Work out the finished part from the listing and answer in its coordinate system (mm). A direction names the side the tool comes from. Round coordinates to 2 decimals unless told otherwise and drop trailing zeros. Loops run counter-clockwise (first coordinate to the right, second up) from the corner with the lowest first, then second, coordinate; pieces in that order, holes last. Notation, with made-up numbers: M 6.25,-2 L 42.25,-2 A25 cw 42.25,20 Z; hole C 58,-17.5 d4. An arc over 180 degrees is marked long. One line per item, written item: value.
```python
from build123d import *

# Parameters (mm, degrees)
F2_SIZE2 = 10
F2_SIZE  = 10
F3_DEPTH = 25
F4_SIZE2 = 12
F4_SIZE  = 12


with BuildPart() as f1:
    # F0 (on Front) → F1 (revolve)
    with BuildSketch(Plane.XZ):
        Polygon((0, 40), (0, 0), (30, 0), (30, 25), (30, 40), align=None)
        with BuildLine():
            Line((30, 25), (30, 0))
            Line((30, 0), (96, 0))
            ThreePointArc((96, 0), (102, 6), (108, 0))
            Line((108, 0), (120, 0))
            Line((120, 0), (120, 25))
            Line((120, 25), (30, 25))
        make_face()
        with BuildLine():
            ThreePointArc((108, 0), (102, 6), (96, 0))
            Line((96, 0), (108, 0))
        make_face()
        with BuildLine():
            Line((108, 0), (96, 0))
            ThreePointArc((96, 0), (102, -6), (108, 0))
        make_face()
    revolve(axis=Axis((75, 0, 0), (1, 0, 0)))

    # F2
    f2_edges = [f1.edges().sort_by_distance(p)[0] for p in [
        (0, 0, -40),
    ]]
    chamfer(f2_edges, length=F2_SIZE, length2=F2_SIZE2)

    # F0 (on Front) → F3 (cut, symmetric)
    with BuildSketch(Plane.XZ):
        with BuildLine():
            ThreePointArc((108, 0), (102, 6), (96, 0))
            Line((96, 0), (108, 0))
        make_face()
        with BuildLine():
            Line((108, 0), (96, 0))
            ThreePointArc((96, 0), (102, -6), (108, 0))
        make_face()
    extrude(amount=F3_DEPTH, both=True, mode=Mode.SUBTRACT)

    # F4
    f4_edges = [f1.edges().sort_by_distance(p)[0] for p in [
        (120, 0, -25),
    ]]
    chamfer(f4_edges, length=F4_SIZE, length2=F4_SIZE2)


solid = f1.part
```
1) Each of these flat-tipped pins is pushed along its axis until it touches: pin 1 (3 mm diameter, centred on x = 105.5, z = 17, fed in from +Y); pin 2 (6 mm diameter, centred on y = 4.5, z = 22, fed in from +X); pin 3 (10 mm diameter, centred on x = 41.5, y = -13.5, fed in from +Z); pin 4 (8 mm diameter, centred on y = 15, z = -0.5, fed in from +X). Where does it stop, or does it pass through?
Check values:
pin 1: y = 19.62
pin 2: x = 113.54
pin 3: z = 23.51
pin 4: x = 120
2) The mould has two halves that part along Z. Classify faces 3 (the face through (0, 0, 0)), 4 (the face through (108, 0, 0)), 5 (the face through (0.49, -9.16, 29.08)): +Z half, -Z half, draft (parallel to the pull), parting line (faces both ways), or undercut.
Check values:
face 3: draft
face 4: undercut
face 5: parting line
3) Find the intervals of material crossed by probe 1 along X at (y, z) = (-1, 0); probe 2 along Z at (x, y) = (104, 20); probe 3 along Z at (x, y) = (102, 1.5), in increasing order. Write a range as from..to.
Check values:
probe 1: 0..96, 108..120
probe 2: -15..-5.66, 5.66..15
probe 3: -24.95..-6, 6..24.95
4) For faces 1 (the face through (19.86, 39.05, -8.67)), 2 (the face through (30, -18.34, -17.22)), determine the directions among +Z, -Z, +X, -X, +Y, -Y from which every point of the face is accessible in a straight line to the end or side of a thin tool.
Check values:
face 1: +X, -X
face 2: +X
5) Find section B-B (x = 88.5). Give the vertices of the cut face in (y, z), then the cut area to 3 significant figures.
Check values:
outline: C 0,0 d50
area: 1,960 mm2
6) Find section A-A (y = 0). Give the vertices of the cut face in (x, z).
Check values:
outline: M 0,-30 L 10,-40 L 30,-40 L 30,-25 L 108,-25 L 120,-13 L 120,13 L 108,25 L 30,25 L 30,40 L 10,40 L 0,30 Z; hole C 102,0 d12
